Geometry: see drawing. Coordinates: mm, zero at the bounding-box minimum. A direction names the side the tool comes from. Round coordinates to 2 decimals unless told otherwise and drop trailing zeros. Loops run counter-clockwise (first coordinate to the right, second up) from the corner with the lowest first, then second, coordinate; pieces in that order, holes last. Notation, with made-up numbers: (-18, 14) -> (4, 14) arc R10 ccw to (4, 19) -> close; hole circle Ø2 at (20.5, 53). An arc over 180 degrees is marked (long way). Answer in a Markdown table with one row per item.
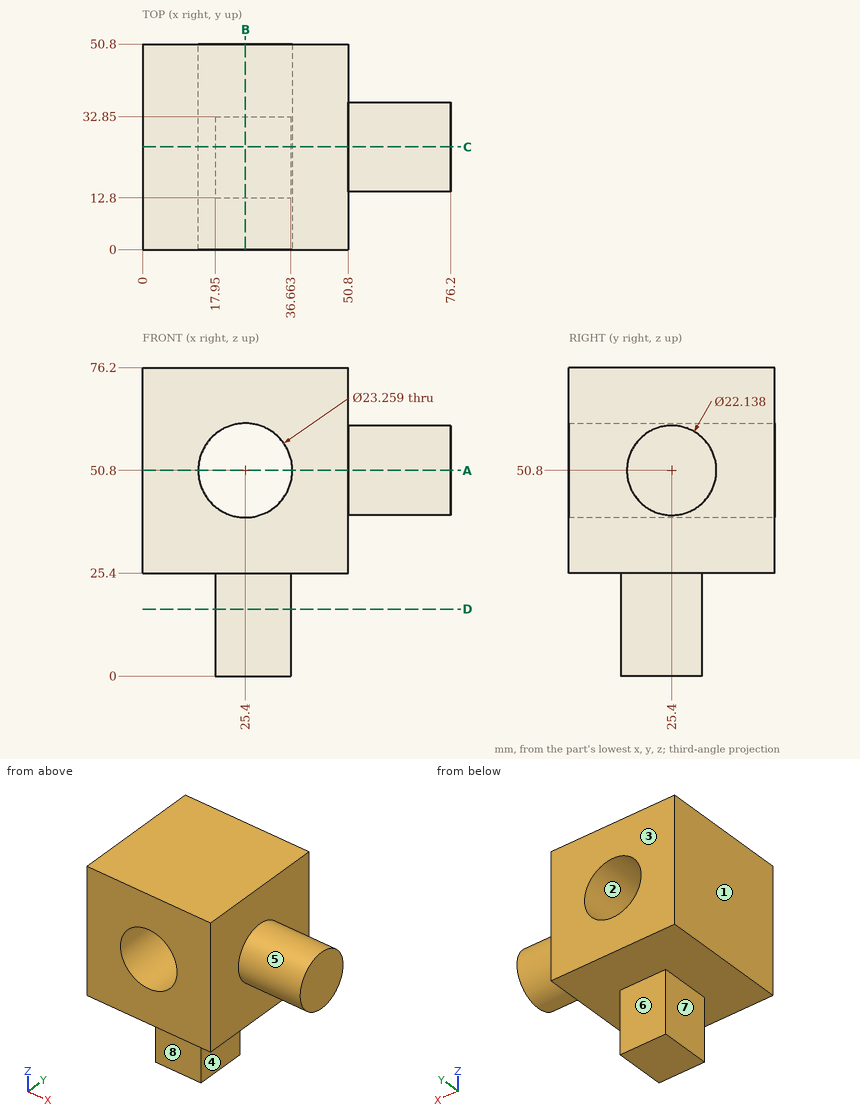
Item 1: Mould query, pull axis X, two halves, no side actions, for the marked faces 1, 2 and 3. Classes: released by +X, released by -X, zero draft, split by the parting line, or undercut.
Ans:
| item | result |
|---|---|
| face 1 | released by -X |
| face 2 | undercut |
| face 3 | zero draft |
Item 2: Section query C-C, the plane y = 25.4. Output: boundary loops of the cut face in (x, z), and give its area (3 significant figures).
Ans:
| item | result |
|---|---|
| outline | (0, 25.4) -> (17.95, 25.4) -> (17.95, 0) -> (36.66, 0) -> (36.66, 25.4) -> (50.8, 25.4) -> (50.8, 39.73) -> (76.2, 39.73) -> (76.2, 61.87) -> (50.8, 61.87) -> (50.8, 76.2) -> (0, 76.2) -> close; hole circle Ø23.26 at (25.4, 50.8) |
| area | 3,190 mm2 |
Item 3: First-contact query: P1, Ø5, axis at y = 32.5, z = 15, coming from the +X side; P2, Ø12, axis at x = 67.5, z = 63.5, coming from the -Y side; P3, Ø9.5, axis at x = 24, z = 11.5, coming from the -Y side. Flat tips, straight axial feed; report the tip coordinate or a pass-through.
Ans:
| item | result |
|---|---|
| P1 | x = 36.66 |
| P2 | y = 16.59 |
| P3 | y = 12.8 |
Item 4: Section query B-B, the plane x = 25.4. Output: boundary loops of the cut face in (y, z), and give its area (3 significant figures).
Ans:
| item | result |
|---|---|
| outline | (0, 25.4) -> (12.8, 25.4) -> (12.8, 0) -> (32.85, 0) -> (32.85, 25.4) -> (50.8, 25.4) -> (50.8, 39.17) -> (0, 39.17) -> close; (0, 62.43) -> (50.8, 62.43) -> (50.8, 76.2) -> (0, 76.2) -> close |
| area | 1,910 mm2 |
Item 5: Ray query, L1, parallel to Z at x = 25, y = 29; L2, parallel to Y at x = 36.5, z = 23; L3, parallel to X at y = 23, z = 23.5. Return the intervals inside material, ascending.
Ans:
| item | result |
|---|---|
| L1 | 0 to 39.18, 62.42 to 76.2 |
| L2 | 12.8 to 32.85 |
| L3 | 17.95 to 36.66 |
Item 6: Set-up query: the marked faces 4, 5, 6, 7 and 8. Return all of +Z, -Z, +X, -X, +Y, -Y with unobstructed straight access to the full face (end or side cutting, diameter ignored); none if empty.
Ans:
| item | result |
|---|---|
| face 4 | -Z, +X, +Y, -Y |
| face 5 | +X |
| face 6 | -Z, +X, -X, +Y |
| face 7 | -Z, -X, +Y, -Y |
| face 8 | -Z, +X, -X, -Y |
Item 7: Section query A-A, the plane z = 50.8. Output: boundary loops of the cut face in (x, y), and give its area (3 significant figures).
Ans:
| item | result |
|---|---|
| outline | (0, 0) -> (13.77, 0) -> (13.77, 50.8) -> (0, 50.8) -> close; (37.03, 0) -> (50.8, 0) -> (50.8, 14.33) -> (76.2, 14.33) -> (76.2, 36.47) -> (50.8, 36.47) -> (50.8, 50.8) -> (37.03, 50.8) -> close |
| area | 1,960 mm2 |
Item 8: Section query D-D, the plane z = 16.5. Output: boundary loops of the cut face in (x, y), and give its area (3 significant figures).
Ans:
| item | result |
|---|---|
| outline | (17.95, 12.8) -> (36.66, 12.8) -> (36.66, 32.85) -> (17.95, 32.85) -> close |
| area | 375 mm2 |
